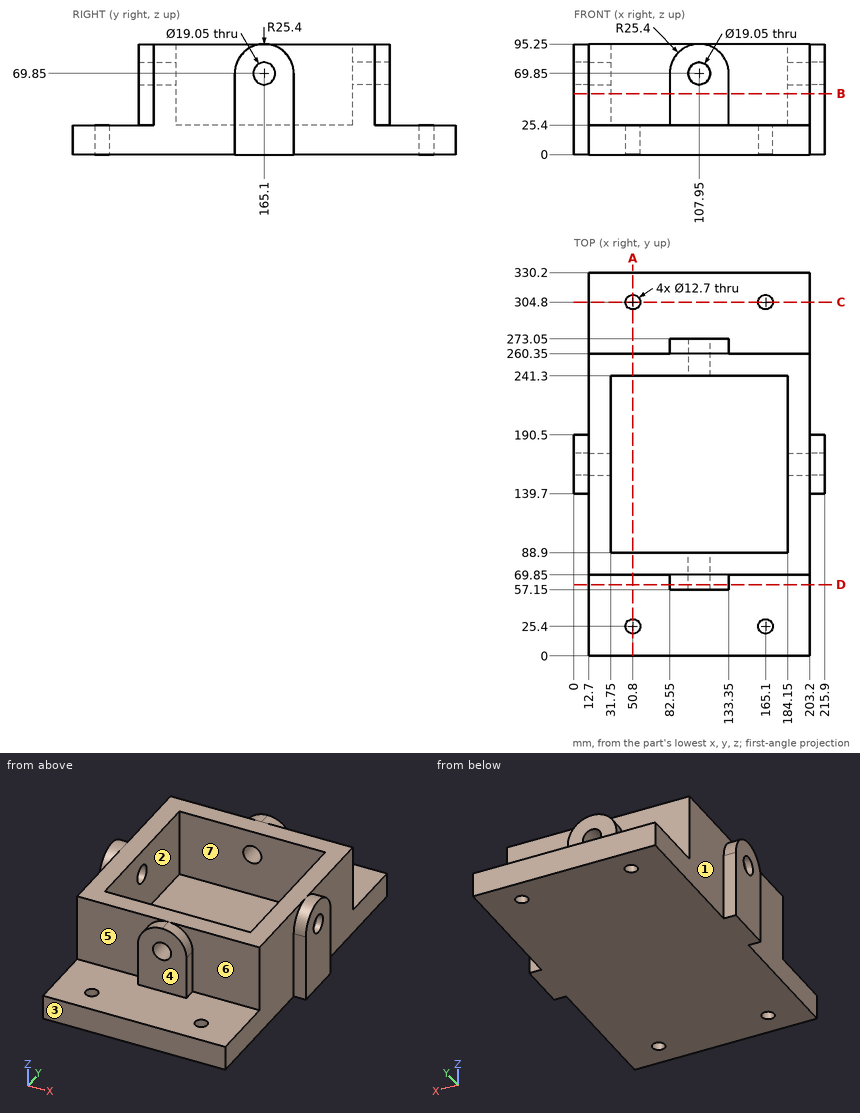
Here's the drawing with two shaded views (mm, measured from the low corner). I have some questions. A direction names the side the tool comes from. Give positions to 0.01 mm unless a question says otherwise; leave off trailing zeros. Loops run counter-clockwise (first coordinate to the right, second up) from the corner with the lowest first, then second, coordinate; pieces in that order, holes last. Notation, with made-up numbers: (76.5, 74) -> (118.5, 74) arc R31 ccw to (118.5, 98) -> close; hole circle Ø10 at (82.25, 2). An arc over 180 degrees is marked (long way). One line per item, written item: value.
Q1. Suppose I cut it at D-D on y = 61.5. Please give me the cut outline in (x, z) (3 decimals), then the cut area to 3 significant figures.
Answers follow:
outline: (12.7, 0) -> (203.2, 0) -> (203.2, 25.4) -> (133.35, 25.4) -> (133.35, 69.85) arc R25.4 ccw to (82.55, 69.85) -> (82.55, 25.4) -> (12.7, 25.4) -> close; hole circle Ø19.05 at (107.95, 69.85)
area: 7,830 mm^2
Q2. If I drill on line 1 along Y through (x, z) = (165.1, 20.25); line 2 along Z through (x, y) = (2, 165); line 3 along Y through (x, z) = (181, 28), over which ranges is the centre line in solid material (lowest first)?
Answers follow:
line 1: 0 to 19.05, 31.75 to 298.45, 311.15 to 330.2
line 2: 0 to 60.33, 79.37 to 95.25
line 3: 69.85 to 88.9, 241.3 to 260.35
Q3. Suppose I cut it at B-B on z = 52.5. Please give me the cut outline in (x, y), then the cut area to 3 significant figures.
Answers follow:
outline: (0, 139.7) -> (12.7, 139.7) -> (12.7, 69.85) -> (82.55, 69.85) -> (82.55, 57.15) -> (133.35, 57.15) -> (133.35, 69.85) -> (203.2, 69.85) -> (203.2, 139.7) -> (215.9, 139.7) -> (215.9, 190.5) -> (203.2, 190.5) -> (203.2, 260.35) -> (133.35, 260.35) -> (133.35, 273.05) -> (82.55, 273.05) -> (82.55, 260.35) -> (12.7, 260.35) -> (12.7, 190.5) -> (0, 190.5) -> close; hole (31.75, 88.9) -> (184.15, 88.9) -> (184.15, 241.3) -> (31.75, 241.3) -> close
area: 15,600 mm^2
Q4. On a 3-axis mill with a long thin cutter (end or side, diameter ignored), from which of +Z, -Z, +X, -X, +Y, -Y can I reach the whole of each face in a straight line? I mean the marked faces 4, 5, 6 and 7. Say none if no direction works.
Answers follow:
face 4: +Z, +X, -X, -Y
face 5: +Z, -X, -Y
face 6: +Z, +X, -Y
face 7: +Z
Q5. We'd pull the mould along X, two halves only. Please class the marked faces 1, 2 and 3: pulls with the +X half, pulls with the -X half, needs draft (parallel to the pull), parting line crosses it, or undercut.
Answers follow:
face 1: pulls with the -X half
face 2: undercut
face 3: needs draft
Q6. I'm going to push flat-ended pins straight in: pin 1 Ø14 at (y, z) = (267.5, 55) entering from +X; pin 2 Ø11.5 at (y, z) = (165.1, 69.85) entering from -X; pin 3 Ø2 at (x, z) = (175.5, 35.5) entering from -Y; pin 4 Ø6.5 at (x, z) = (7.5, 45) entering from -Y. Where does each tip first touch, or does it pass through?
Answers follow:
pin 1: x = 133.35
pin 2: through
pin 3: y = 69.85
pin 4: y = 139.7
Q7. Suppose I cut it at C-C on y = 304.8. Please give me the cut outline in (x, z), then the cut area to 3 significant figures.
Answers follow:
outline: (12.7, 0) -> (44.45, 0) -> (44.45, 25.4) -> (12.7, 25.4) -> close; (57.15, 0) -> (158.75, 0) -> (158.75, 25.4) -> (57.15, 25.4) -> close; (171.45, 0) -> (203.2, 0) -> (203.2, 25.4) -> (171.45, 25.4) -> close
area: 4,190 mm^2
Q8. Suppose I cut it at A-A on x = 50.8. Please give me the cut outline in (y, z).
Answers follow:
outline: (0, 0) -> (19.05, 0) -> (19.05, 25.4) -> (0, 25.4) -> close; (31.75, 0) -> (298.45, 0) -> (298.45, 25.4) -> (260.35, 25.4) -> (260.35, 95.25) -> (241.3, 95.25) -> (241.3, 25.4) -> (88.9, 25.4) -> (88.9, 95.25) -> (69.85, 95.25) -> (69.85, 25.4) -> (31.75, 25.4) -> close; (311.15, 0) -> (330.2, 0) -> (330.2, 25.4) -> (311.15, 25.4) -> close
